Verification items for the finished model (mm, model axes). Coordinates: 2 decimals unless noted, no trailing zeros. Order: outer loops, then holes, each group sorted by start corner. A loop starts at its lowest first (then second) coordinate and runs counter-clockwise, first axis right, second up. Notation, with made-up numbers: M 40.5,31.25 L 54.5,31.25 A19 cw 54.5,62.25 Z; hole C -25.5,-28 d10. An arc over 180 degrees is marked long. Return JSON: item names as keys, results as strings. Group by question number.
1. Section check D-D, the plane x = 77.5. Record the cut outline in (y, z), plus the area to 3 significant figures.
2. Section check C-C, the plane z = 3.25. Record the cut outline in (x, y), plus the area to 3 significant figures.
3. Mould release check, pull along Y, two halves, no side actions. Record for faces 1 (the flat face through (24, 16, 5)), 2 (the cylindrical face through (18, 89, 2)), 3 (the cylindrical face through (52, 10, 2)): +Y half, -Y half, draft (parallel to the pull), parting line (faces both ways), or undercut.
4. Section check A-A, the plane y = 10. Record the cut outline in (x, z).
5. Material ranges on line 1 along Y through (x, z) = (10, 3.95); line 2 along Y through (x, z) = (55, 1.65), recorded low to high.
6. Gauge pin test, flat ends, axial feed: pin 1 (5 mm diameter, centred on x = 55, y = 10, fed in from -Z); pin 2 (1 mm diameter, centred on x = 21.5, y = 13.5, fed in from -Z); pin 3 (1.5 mm diameter, centred on x = 61.5, z = 2, fed in from +Y). Record the tip position at first contact, or that the pin passes through.
```python
from build123d import *

# Parameters (mm, degrees)
SKETCH_W        = 90
SKETCH_H        = 90
PAD_DEPTH       = 5
SKETCH001_W     = 90
SKETCH001_H     = 90
POCKET_DEPTH    = 5
SKETCH002_R     = 5
POCKET001_DEPTH = 5
FILLET_R        = 5
SKETCH003_R     = 3
POCKET002_DEPTH = 5


with BuildPart() as part:
    # Sketch → Pad (new body)
    with BuildSketch(Plane.XY):
        with Locations((45, 45)):
            Rectangle(SKETCH_W, SKETCH_H)
    extrude(amount=PAD_DEPTH)

    # Sketch001 (on Face6 of Pad) → Pocket (cut)
    with BuildSketch(Plane.XY.offset(5)):
        with Locations((65, 65)):
            Rectangle(SKETCH001_W, SKETCH001_H)
    extrude(amount=-POCKET_DEPTH, mode=Mode.SUBTRACT)

    # Sketch002 (on Face4 of Pocket) → Pocket001 (cut)
    with BuildSketch(Plane.XY.offset(5)):
        with Locations((20, 20)):
            Circle(SKETCH002_R)
    extrude(amount=-POCKET001_DEPTH, mode=Mode.SUBTRACT)

    # Fillet
    fillet_edges = [part.edges().sort_by_distance(p)[0] for p in [
        (20, 25, 2.5),
        (25, 20, 2.5),
        (0, 0, 2.5),
        (90, 20, 2.5),
        (90, 0, 2.5),
        (20, 90, 2.5),
        (0, 90, 2.5),
    ]]
    fillet(fillet_edges, radius=FILLET_R)

    # Sketch003 (on Face2 of Fillet) → Pocket002 (cut)
    with BuildSketch(Plane(origin=(0, 0, 0), x_dir=(1, 0, 0), z_dir=(0, 0, -1))):
        with Locations((32.5, -10)):
            Circle(SKETCH003_R)
        with Locations((55, -10)):
            Circle(SKETCH003_R)
        with Locations((77.5, -10)):
            Circle(SKETCH003_R)
        with Locations((10, -32.5)):
            Circle(SKETCH003_R)
        with Locations((10, -55)):
            Circle(SKETCH003_R)
        with Locations((10, -77.5)):
            Circle(SKETCH003_R)
        with Locations((10, -10)):
            Circle(SKETCH003_R)
    extrude(amount=-POCKET002_DEPTH, mode=Mode.SUBTRACT)


solid = part.part
```
Answers follow:
{
 "1": {"outline": "M 0,0 L 7,0 L 7,5 L 0,5 Z; M 13,0 L 20,0 L 20,5 L 13,5 Z", "area": "70.0 mm^2"},
 "2": {"outline": "M 0,5 A5 ccw 5,0 L 85,0 A5 ccw 90,5 L 90,15 A5 ccw 85,20 L 28.66,20 A5 ccw 24.33,17.5 A5 cw long 17.5,24.33 A5 ccw 20,28.66 L 20,85 A5 ccw 15,90 L 5,90 A5 ccw 0,85 Z; hole C 10,10 d6; hole C 10,32.5 d6; hole C 10,55 d6; hole C 10,77.5 d6; hole C 32.5,10 d6; hole C 55,10 d6; hole C 77.5,10 d6", "area": "2,910 mm^2"},
 "3": {"face 1": "draft", "face 2": "+Y half", "face 3": "undercut"},
 "4": {"outline": "M 0,0 L 7,0 L 7,5 L 0,5 Z; M 13,0 L 29.5,0 L 29.5,5 L 13,5 Z; M 35.5,0 L 52,0 L 52,5 L 35.5,5 Z; M 58,0 L 74.5,0 L 74.5,5 L 58,5 Z; M 80.5,0 L 90,0 L 90,5 L 80.5,5 Z"},
 "5": {"line 1": "0 to 7, 13 to 29.5, 35.5 to 52, 58 to 74.5, 80.5 to 90", "line 2": "0 to 7, 13 to 20"},
 "6": {"pin 1": "through", "pin 2": "z = 0", "pin 3": "y = 20"}
}
